Here's the drawing with two shaded views (mm, measured from the low corner). I have some questions. Give positions to 0.01 mm unless a question says otherwise; leave off trailing zeros. Loops run counter-clockwise (first coordinate to the right, second up) from the corner with the lowest first, then second, coordinate; pieces in that order, holes last. Notation, with made-up numbers: (74, 49) -> (87, 49) arc R15 ccw to (87, 64) -> close; hole circle Ø9 at (16, -25.5). An arc over 180 degrees is marked (long way). Answer in a Markdown table with one row per item. Add a question column.
Item 1: If we section it at C-C (z = 1.8): Write out the boundary of the cut face in (x, y).
Item 2: For P1, Ø1.5, axis at y = 56, z = 0.5, coming from the -X side; P2, Ø6.5, axis at x = 7, y = 63, coming from the -Z side, each with a flat end and sliding along its axis, tell me the tip position at first contact or that it passes through.
Item 3: If I drill on line 1 (Y direction, x = 7, z = 1.4); line 2 (Y direction, x = 61, z = 2.1), over which ranges is the centre line in solid material (lowest first)?
Item 4: If we section it at A-A (x = 7): Write out the boundary of the cut face in (y, z), then the cut area to 3 significant figures.
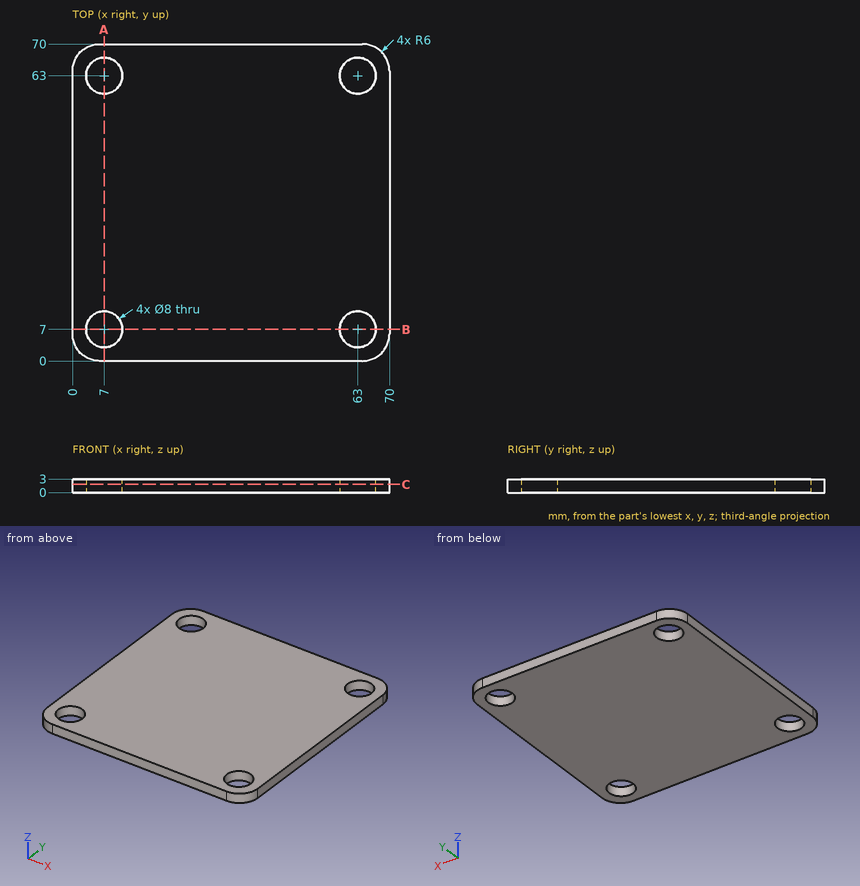
Recorded:
| question | item | result |
|---|---|---|
| 1 | outline | (0, 6) arc R6 ccw to (6, 0) -> (64, 0) arc R6 ccw to (70, 6) -> (70, 64) arc R6 ccw to (64, 70) -> (6, 70) arc R6 ccw to (0, 64) -> close; hole circle Ø8 at (7, 7); hole circle Ø8 at (7, 63); hole circle Ø8 at (63, 7); hole circle Ø8 at (63, 63) |
| 2 | P1 | stops at x = 0 |
| 2 | P2 | passes through |
| 3 | line 1 | y = 0 to 3, 11 to 59, 67 to 70 |
| 3 | line 2 | y = 0 to 3.54, 10.46 to 59.54, 66.46 to 70 |
| 4 | outline | (0, 0) -> (3, 0) -> (3, 3) -> (0, 3) -> close; (11, 0) -> (59, 0) -> (59, 3) -> (11, 3) -> close; (67, 0) -> (70, 0) -> (70, 3) -> (67, 3) -> close |
| 4 | area | 162 mm^2 |
